Input: part model. Units: mm. Frame: model coordinates. Give positions to 0.01 mm unless a question says otherwise; leave off trailing zeros. Order: outer loops, then holes, each group sorted by start corner. A loop starts at its lowest first (then second) coordinate and runs counter-clockwise, first axis right, second up. Notation, with made-up numbers: M -12.5,41 L 9.5,41 A13 ccw 9.5,66 Z; hole C 4,76.25 d10. An arc over 180 degrees is marked long. Use a Markdown table: item, result.
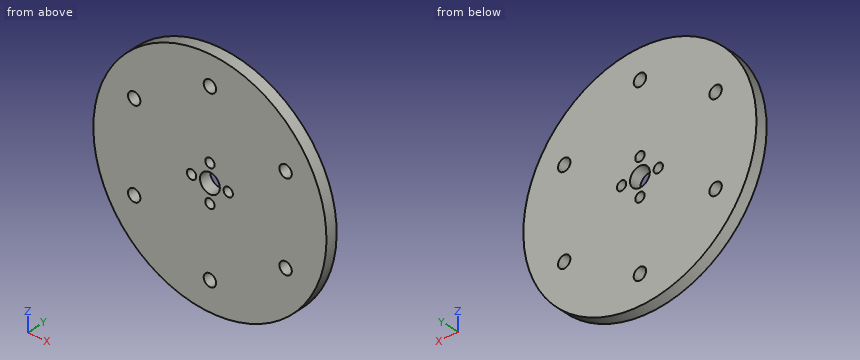
from build123d import *

# Parameters (mm, degrees)
SKETCH1_R           = 50.8
BOSS_EXTRUDE1_DEPTH = 5.08
SKETCH2_R           = 2.69875
CUT_EXTRUDE1_DEPTH  = 5.08
SKETCH3_R           = 4.318
SKETCH3_R_2         = 2.032
CUT_EXTRUDE2_DEPTH  = 5.08


with BuildPart() as part:
    # Sketch1 → Boss-Extrude1 (new body)
    with BuildSketch(Plane(origin=(0, 0, 0), x_dir=(1, 0, 0), z_dir=(0, 1, 0))):
        with Locations(Location((0, 0, 0), (0, 0, 270))):
            Circle(SKETCH1_R)
    extrude(amount=BOSS_EXTRUDE1_DEPTH)

    # Sketch2 → Cut-Extrude1 (cut)
    with BuildSketch(Plane(origin=(0, 5.08, 0), x_dir=(1, 0, 0), z_dir=(0, 1, 0))):
        with Locations(Location((0, -38.1, 0), (0, 0, 270))):
            Circle(SKETCH2_R)
        with Locations(Location((-32.995567884, -19.05, 0), (0, 0, 270))):
            Circle(SKETCH2_R)
        with Locations(Location((-32.995567884, 19.05, 0), (0, 0, 270))):
            Circle(SKETCH2_R)
        with Locations(Location((0, 38.1, 0), (0, 0, 270))):
            Circle(SKETCH2_R)
        with Locations(Location((32.995567884, 19.05, 0), (0, 0, 270))):
            Circle(SKETCH2_R)
        with Locations(Location((32.995567884, -19.05, 0), (0, 0, 270))):
            Circle(SKETCH2_R)
    extrude(amount=-CUT_EXTRUDE1_DEPTH, mode=Mode.SUBTRACT)

    # Sketch3 → Cut-Extrude2 (cut)
    with BuildSketch(Plane.XZ):
        with Locations(Location((0, 0, 0), (0, 0, 270))):
            Circle(SKETCH3_R)
        with Locations(Location((0, -8.001, 0), (0, 0, 270))):
            Circle(SKETCH3_R_2)
        with Locations(Location((-8.001, 0, 0), (0, 0, 270))):
            Circle(SKETCH3_R_2)
        with Locations(Location((0, 8.001, 0), (0, 0, 270))):
            Circle(SKETCH3_R_2)
        with Locations(Location((8.001, 0, 0), (0, 0, 270))):
            Circle(SKETCH3_R_2)
    extrude(amount=-CUT_EXTRUDE2_DEPTH, mode=Mode.SUBTRACT)


solid = part.part
1) First-contact query: pin 1 Ø3 at (x, y) = (13, 3) entering from +Z; pin 2 Ø2.5 at (x, z) = (0, -8.001) entering from -Y; pin 3 Ø1.5 at (x, y) = (4, 2.5) entering from +Z. Flat tips, straight axial feed; report the tip coordinate or a pass-through.
Response values:
| item | result |
|---|---|
| pin 1 | stops at z = 49.48 |
| pin 2 | passes through |
| pin 3 | stops at z = 50.7 |
2) Cut plane B-B on z = 19.05. Return loops of the section in (x, y), and give its area (3 significant figures).
Response values:
| item | result |
|---|---|
| outline | M -47.09,0 L -35.69,0 L -35.69,5.08 L -47.09,5.08 Z; M -30.3,0 L 30.3,0 L 30.3,5.08 L -30.3,5.08 Z; M 35.69,0 L 47.09,0 L 47.09,5.08 L 35.69,5.08 Z |
| area | 424 mm² |
3) Cut plane D-D on y = 0.95. State how many separate pieces and enclosed holes the cut face has, and give its area (3 significant figures).
Response values:
| item | result |
|---|---|
| separate pieces | 1 |
| enclosed holes | 11 |
| area | 7,860 mm² |
4) Cut plane C-C on z = -8. Return loops of the section in (x, y).
Response values:
| item | result |
|---|---|
| outline | M -50.17,0 L -2.03,0 L -2.03,5.08 L -50.17,5.08 Z; M 2.03,0 L 50.17,0 L 50.17,5.08 L 2.03,5.08 Z |
5) Material intervals for line 1 (X direction, y = 2.5, z = 0); line 2 (X direction, y = 2.8, z = 19.05); line 3 (Z direction, x = 32.5, y = 4.75), sorted ascending. Write a range as from..to.
Response values:
| item | result |
|---|---|
| line 1 | x = -50.8..-10.03, -5.97..-4.32, 4.32..5.97, 10.03..50.8 |
| line 2 | x = -47.09..-35.69, -30.3..30.3, 35.69..47.09 |
| line 3 | z = -39.04..-21.7, -16.4..16.4, 21.7..39.04 |
6) Cut plane A-A on x = 0. Return loops of the section in (y, z), and give its area (3 significant figures).
Response values:
| item | result |
|---|---|
| outline | M 0,-50.8 L 5.08,-50.8 L 5.08,-40.8 L 0,-40.8 Z; M 0,-35.4 L 5.08,-35.4 L 5.08,-10.03 L 0,-10.03 Z; M 0,-5.97 L 5.08,-5.97 L 5.08,-4.32 L 0,-4.32 Z; M 0,4.32 L 5.08,4.32 L 5.08,5.97 L 0,5.97 Z; M 0,10.03 L 5.08,10.03 L 5.08,35.4 L 0,35.4 Z; M 0,40.8 L 5.08,40.8 L 5.08,50.8 L 0,50.8 Z |
| area | 376 mm² |
